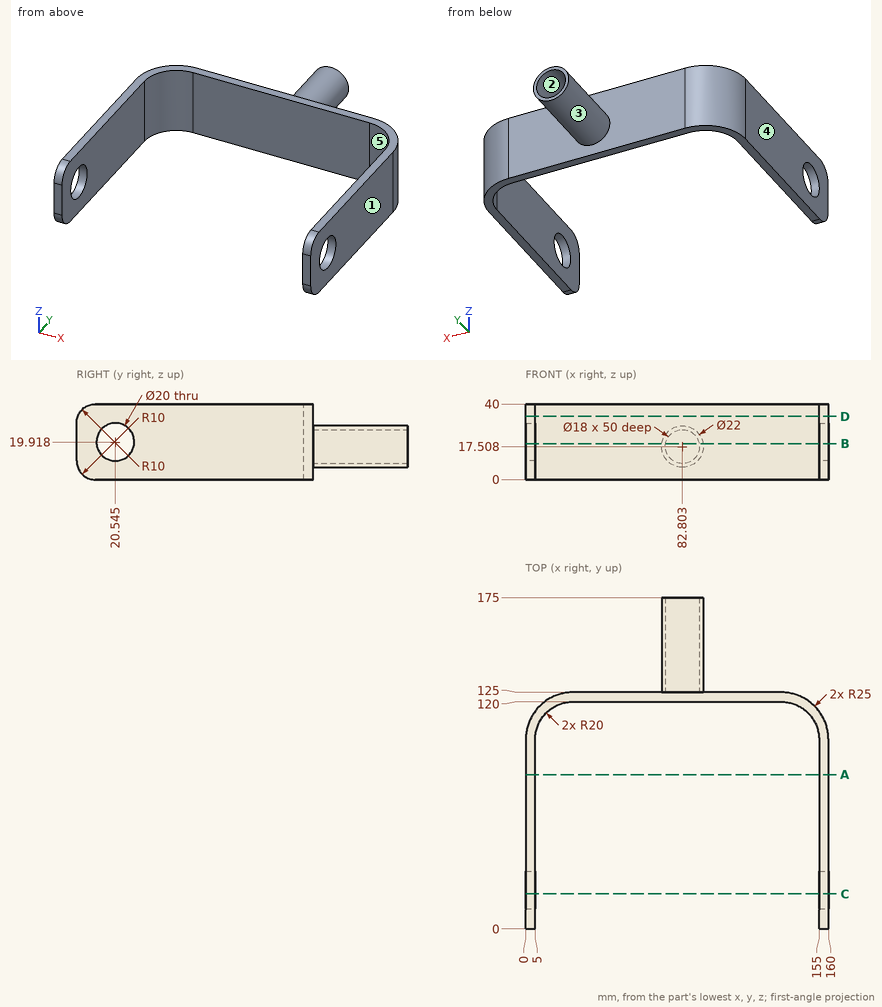
Source: three-view drawing plus pictorial views. Frame: mm from the lowest corner of the part. A direction names the side the tool comes from. Coordinates: 2 decimals unless noted, no trailing zeros. Write each loop counter-clockwise with the first axis right and the second up, starting at its lowest first coordinate (ties: lowest second). Pieces come first, ordered by that corner, then holes. Notation, with made-up numbers: (42.25, 80.25) - (55.25, 80.25) arc R4 ccw to (55.25, 86.25) - close; hole circle Ø3 at (-22.5, 45). An arc over 180 degrees is marked (long way). Return JSON: item names as keys, results as strings.
Item 1: Section query A-A (y = 81.5). Output: boundary loops of the cut face in (x, z), and give its area (3 significant figures).
Completed:
{"outline": "(0, 0) - (5, 0) - (5, 40) - (0, 40) - close; (155, 0) - (160, 0) - (160, 40) - (155, 40) - close", "area": "400 mm2"}
Item 2: Section query B-B (z = 19). Output: boundary loops of the cut face in (x, y) (1 decimal), and give its area (3 significant figures).
Completed:
{"outline": "(0, 0) - (5, 0) - (5, 10.6) - (0, 10.6) - close; (0, 30.5) - (5, 30.5) - (5, 100) arc R20 cw to (25, 120) - (135, 120) arc R20 cw to (155, 100) - (155, 30.5) - (160, 30.5) - (160, 100) arc R25 ccw to (135, 125) - (93.7, 125) - (93.7, 175) - (91.7, 175) - (91.7, 125) - (73.9, 125) - (73.9, 175) - (71.9, 175) - (71.9, 125) - (25, 125) arc R25 ccw to (0, 100) - close; (155, 0) - (160, 0) - (160, 10.6) - (155, 10.6) - close", "area": "1,910 mm2"}
Item 3: Pin query (flat end, axial travel): pin 1 Ø20 at (x, z) = (56, 12.5) entering from -Y; pin 2 Ø1.5 at (x, z) = (27, 22) entering from +Y. Return the tip coordinate at first contact, or that it passes through.
Completed:
{"pin 1": "stops at y = 120", "pin 2": "stops at y = 125"}
Item 4: Section query D-D (z = 33.5). Output: boundary loops of the cut face in (x, y).
Completed:
{"outline": "(0, 0.63) - (5, 0.63) - (5, 100) arc R20 cw to (25, 120) - (135, 120) arc R20 cw to (155, 100) - (155, 0.63) - (160, 0.63) - (160, 100) arc R25 ccw to (135, 125) - (25, 125) arc R25 ccw to (0, 100) - close"}
Item 5: Pull-direction query (Z, two-part tool) for the marked faces 1, 2 and 3; classes: +Z half, -Z half, draft (parallel to the pull), parting line (faces both ways), or undercut.
Completed:
{"face 1": "draft", "face 2": "undercut", "face 3": "parting line"}
Item 6: Reachability of the marked faces 4 and 5 from +Z, -Z, +X, -X, +Y, -Y: full face, straight path, thin tool, end or side. Return the list, or none.
Completed:
{"face 4": "+Z, -Z, -X, +Y, -Y", "face 5": "+Z, -Z, -Y"}
Item 7: Section query C-C (y = 18.5). Output: boundary loops of the cut face in (x, z).
Completed:
{"outline": "(0, 0) - (5, 0) - (5, 10.13) - (0, 10.13) - close; (0, 29.71) - (5, 29.71) - (5, 40) - (0, 40) - close; (155, 0) - (160, 0) - (160, 10.13) - (155, 10.13) - close; (155, 29.71) - (160, 29.71) - (160, 40) - (155, 40) - close"}
Item 8: Line query: L1, parallel to X at y = 47, z = 13.5; L2, parallel to Y at x = 135.5, z = 11 (1 decimal); L3, parallel to X at y = 140, z = 12 (1 decimal). Output: solid intervals per line, ascending.
Completed:
{"L1": "x = 0 to 5, 155 to 160", "L2": "y = 120 to 125", "L3": "x = 73.3 to 75.7, 89.9 to 92.3"}
